from build123d import *

# Parameters (mm, degrees)
SKETCH1_R            = 1.75
BOSS_EXTRUDE1_DEPTH  = 9
SHELL2_START         = 2.55
SHELL2_OUTLINE_W     = 24.9
SHELL2_OUTLINE_H     = 24.9
SHELL2_DEPTH         = 6.45
CUT_EXTRUDE1_REACH   = 27.052
SKETCH6_R            = 11.5
BOSS_EXTRUDE5_DEPTH  = 25
SHELL7_T             = -1
CUT_EXTRUDE6_START   = -1
SKETCH12_R           = 11.5
CUT_EXTRUDE6_DEPTH   = 1
SKETCH19_W           = 3
SKETCH19_H           = 25.5
BOSS_EXTRUDE17_DEPTH = 23
SKETCH20_W           = 3
SKETCH20_H           = 25.5
BOSS_EXTRUDE18_DEPTH = 23
SKETCH21_W           = 79
SKETCH21_H           = 55
SKETCH21_W_2         = 76
SKETCH21_H_2         = 25.5
BOSS_EXTRUDE19_DEPTH = 3
FILLET1_R            = 3
SKETCH22_R           = 2.0955
CUT_EXTRUDE7_DEPTH   = 3
BOSS_EXTRUDE34_REACH = 56.236
SKETCH37_R           = 2.5146
CUT_EXTRUDE8_DEPTH   = 1.27


# Read off the part's stored shape, not the designer's step: Shell2
with BuildPart() as part:
    # Sketch1 → Boss-Extrude1 (new body)
    with BuildSketch(Plane.XY):
        with BuildLine():
            Line((15, 15), (4, 15))
            ThreePointArc((4, 15), (0, 19), (-4, 15))
            Line((-4, 15), (-15, 15))
            Line((-15, 15), (-15, -15))
            Line((-15, -15), (-4, -15))
            ThreePointArc((-4, -15), (0, -19), (4, -15))
            Line((4, -15), (15, -15))
            Line((15, -15), (15, 15))
        make_face()
        with Locations((0, -15)):
            Circle(SKETCH1_R, mode=Mode.SUBTRACT)
        with Locations((0, 15)):
            Circle(SKETCH1_R, mode=Mode.SUBTRACT)
    extrude(amount=BOSS_EXTRUDE1_DEPTH)

    # Shell2 outline → Shell2 (cut)
    with BuildSketch(Plane.XY.offset(SHELL2_START)):
        Rectangle(SHELL2_OUTLINE_W, SHELL2_OUTLINE_H)
    extrude(amount=SHELL2_DEPTH, mode=Mode.SUBTRACT)

    # Sketch6 → Cut-Extrude1 (cut, up to next)
    with BuildSketch(Plane.XY.offset(2.55), mode=Mode.PRIVATE) as cut_extrude1_sk1:
        Circle(SKETCH6_R)
    cut_extrude1_tool1 = extrude(cut_extrude1_sk1.sketch, amount=-CUT_EXTRUDE1_REACH, mode=Mode.PRIVATE) & part.part
    add(cut_extrude1_tool1.solids().sort_by_distance((0, 0, 2.55))[0], mode=Mode.SUBTRACT)


with BuildPart() as body_2:
    # Sketch11 → Boss-Extrude5 (new body)
    with BuildSketch(Plane(origin=(0, 0, 0), x_dir=(-1, 0, 0), z_dir=(0, 0, -1))):
        Polygon((-15, -12.75), (2.39, -12.75), (15, -12.75), (15, 12.75), (2.39, 12.75), (-15, 12.75), align=None)
    extrude(amount=BOSS_EXTRUDE5_DEPTH)

    # Shell7
    shell7_openings = [body_2.faces().sort_by_distance(p)[0] for p in [
        (0, 0, -25),
    ]]
    offset(amount=SHELL7_T, openings=shell7_openings, kind=Kind.INTERSECTION)

    # Sketch12 → Cut-Extrude6 (cut)
    with BuildSketch(Plane(origin=(0, 0, -1), x_dir=(-1, 0, 0), z_dir=(0, 0, -1)).offset(CUT_EXTRUDE6_START)):
        with Locations(Location((0, 0, 0), (0, 0, 180))):
            Circle(SKETCH12_R)
    extrude(amount=CUT_EXTRUDE6_DEPTH, mode=Mode.SUBTRACT)

    # Sketch19 → Boss-Extrude17 (add)
    with BuildSketch(Plane(origin=(15, 0, 0), x_dir=(0, 0, -1), z_dir=(1, 0, 0))):
        with Locations((23.5, 0)):
            Rectangle(SKETCH19_W, SKETCH19_H)
    extrude(amount=BOSS_EXTRUDE17_DEPTH)

    # Sketch20 → Boss-Extrude18 (add)
    with BuildSketch(Plane.ZY.offset(15)):
        with Locations((-23.5, 0)):
            Rectangle(SKETCH20_W, SKETCH20_H)
    extrude(amount=BOSS_EXTRUDE18_DEPTH)

    # Sketch21 → Boss-Extrude19 (add)
    with BuildSketch(Plane(origin=(0, 0, -25), x_dir=(-1, 0, 0), z_dir=(0, 0, -1))):
        Rectangle(SKETCH21_W, SKETCH21_H)
        Rectangle(SKETCH21_W_2, SKETCH21_H_2, mode=Mode.SUBTRACT)
    extrude(amount=-BOSS_EXTRUDE19_DEPTH)

    # Fillet1
    fillet1_edges = [body_2.edges().sort_by_distance(p)[0] for p in [
        (-39.5, -27.5, -23.5),
        (39.5, -27.5, -23.5),
        (39.5, 27.5, -23.5),
        (-39.5, 27.5, -23.5),
    ]]
    fillet(fillet1_edges, radius=FILLET1_R)

    # Sketch22 → Cut-Extrude7 (cut)
    with BuildSketch(Plane(origin=(0, 0, -25), x_dir=(-1, 0, 0), z_dir=(0, 0, -1))):
        with Locations((-27.34, 0)):
            Circle(SKETCH22_R)
        with Locations((27.34, 0)):
            Circle(SKETCH22_R)
    extrude(amount=-CUT_EXTRUDE7_DEPTH, mode=Mode.SUBTRACT)

    # Sketch31 → Boss-Extrude34 (add, up to next)
    with BuildSketch(Plane(origin=(0, 0, 0), x_dir=(-1, 0, 0), z_dir=(0, 0, -1)), mode=Mode.PRIVATE) as boss_extrude34_sk1:
        with BuildLine():
            Line((15, 15), (4, 15))
            ThreePointArc((4, 15), (0, 19), (-4, 15))
            Line((-4, 15), (-15, 15))
            Line((-15, 15), (-15, 12.75))
            Line((-15, 12.75), (15, 12.75))
            Line((15, 12.75), (15, 15))
        make_face()
    boss_extrude34_tool1 = extrude(boss_extrude34_sk1.sketch, amount=BOSS_EXTRUDE34_REACH, mode=Mode.PRIVATE) - body_2.part
    # Sketch31 → Boss-Extrude34 (add, up to next)
    with BuildSketch(Plane(origin=(0, 0, 0), x_dir=(-1, 0, 0), z_dir=(0, 0, -1)), mode=Mode.PRIVATE) as boss_extrude34_sk2:
        with BuildLine():
            Line((15, -12.75), (-15, -12.75))
            Line((-15, -12.75), (-15, -15))
            Line((-15, -15), (-4, -15))
            ThreePointArc((-4, -15), (0, -19), (4, -15))
            Line((4, -15), (15, -15))
            Line((15, -15), (15, -12.75))
        make_face()
    boss_extrude34_tool2 = extrude(boss_extrude34_sk2.sketch, amount=BOSS_EXTRUDE34_REACH, mode=Mode.PRIVATE) - body_2.part

    add(part.part)  # Boss-Extrude34 merges part
    add(boss_extrude34_tool1.solids().sort_by_distance((0, 14.640831, 0))[0])
    add(boss_extrude34_tool2.solids().sort_by_distance((0, -14.640831, 0))[0])

    # Sketch37 → Cut-Extrude8 (cut)
    with BuildSketch(Plane.XY.offset(9)):
        with Locations((0, 15)):
            Circle(SKETCH37_R)
        with Locations((0, -15)):
            Circle(SKETCH37_R)
    extrude(amount=-CUT_EXTRUDE8_DEPTH, mode=Mode.SUBTRACT)


solid = body_2.part
Input: part model. Units: mm. Frame: model coordinates. A direction names the side the tool comes from. Coordinates: 2 decimals unless noted, no trailing zeros. Loops run counter-clockwise (first coordinate to the right, second up) from the corner with the lowest first, then second, coordinate; pieces in that order, holes last.
(1) Material intervals for probe 1 along X at (y, z) = (-0.5, 2); probe 2 along X at (y, z) = (-4, -10.5); probe 3 along Y at (x, z) = (5, -4), sorted ascending.
(2) Set-up query: faces 1 (the face through (0, 11.75, -13)), 2 (the face through (9, -15, -7)), 3 (the face through (15, 0, -6)), 4 (the face through (0, -19, -7)), 5 (the face through (-2, -16, 7.73)). Return all of +Z, -Z, +X, -X, +Y, -Y with unobstructed straight access to the full face (end or side cutting, diameter ignored); none if empty.
(3) Section A-A on z = -15. Return the cut outline in (x, y), then the cut area to 3 significant figures.
(4) First-contact query: pin 1 Ø5 at (x, y) = (7.5, 19.5) entering from +Z; pin 2 Ø4 at (y, z) = (-18.5, -18) entering from -X; pin 3 Ø7 at (y, z) = (5, 6.5) entering from +X; pin 4 Ø18.5 at (x, y) = (0, 0) entering from +Z. Flat tips, straight axial feed; report the tip coordinate or a pass-through.
(5) Section B-B on x = -27.34. Return the cut outline in (y, z), then the cut area to 3 significant figures.
(6) Pull-direction query (Y, two-part tool) for faces 6 (the face through (0, 12.45, 6)), 7 (the face through (6, -10, -1)), 8 (the face through (-15, 0, -6)), 9 (the face through (38.64, -26.6, -23.48)); classes: released by +Y, released by -Y, zero draft, split by the parting line, or undercut.
(7) Section C-C on y = 3. Return the cut outline in (x, z).
(8) Section D-D on x = 22. Return the cut outline in (y, z), then the cut area to 3 significant figures.
Data:
1. probe 1: x = -15 to -11.49, 11.49 to 15
1. probe 2: x = -15 to -14, 14 to 15
1. probe 3: y = -15 to -11.75, 11.75 to 15
2. face 1: -Z
2. face 2: +Z, +X, -Y
2. face 3: +Z, +X, +Y, -Y
2. face 4: +Z, -Y
2. face 5: +Z
3. outline: (-15, -15) - (-4, -15) arc R4 ccw to (4, -15) - (15, -15) - (15, 15) - (4, 15) arc R4 ccw to (-4, 15) - (-15, 15) - close; hole (-14, -11.75) - (14, -11.75) - (14, 11.75) - (-14, 11.75) - close
3. area: 292 mm2
4. pin 1: stops at z = -22
4. pin 2: stops at x = -3.71
4. pin 3: stops at x = 15
4. pin 4: passes through
5. outline: (-27.5, -25) - (-2.1, -25) - (-2.1, -22) - (-27.5, -22) - close; (2.1, -25) - (27.5, -25) - (27.5, -22) - (2.1, -22) - close
5. area: 152 mm2
6. face 6: undercut
6. face 7: undercut
6. face 8: zero draft
6. face 9: released by -Y
7. outline: (-39.5, -25) - (-14, -25) - (-14, -1) - (-11.1, -1) - (-11.1, 2.55) - (-12.45, 2.55) - (-12.45, 9) - (-15, 9) - (-15, -22) - (-39.5, -22) - close; (11.1, -1) - (14, -1) - (14, -25) - (39.5, -25) - (39.5, -22) - (15, -22) - (15, 9) - (12.45, 9) - (12.45, 2.55) - (11.1, 2.55) - close
8. outline: (-27.5, -25) - (27.5, -25) - (27.5, -22) - (-27.5, -22) - close
8. area: 165 mm2
